```python
from build123d import *

# Parameters (mm, degrees)
BOSS_EXTRUDE1_DEPTH      = 36
BOSS_EXTRUDE1_DEPTH_BACK = 50.5
SKETCH1_R                = 12
SKETCH6_R                = 22.5
BOSS_EXTRUDE6_DEPTH      = 10.5
BOSS_EXTRUDE7_START      = 10
SKETCH7_R                = 22.5
BOSS_EXTRUDE7_DEPTH      = 10
SKETCH2_R                = 6.75
BOSS_EXTRUDE2_DEPTH      = 12
SKETCH3_R                = 107.5
BOSS_EXTRUDE3_DEPTH      = 10
SKETCH5_R                = 15
BOSS_EXTRUDE5_DEPTH      = 5
SKETCH4_R                = 6.75
BOSS_EXTRUDE4_DEPTH      = 12


with BuildPart() as part:
    # Sketch1 → Boss-Extrude1 (new, two sides: drawn at the far end of the back side and taken through both)
    with BuildSketch(Plane.XY.offset(-BOSS_EXTRUDE1_DEPTH_BACK)):
        Circle(SKETCH1_R)
    extrude(amount=BOSS_EXTRUDE1_DEPTH + BOSS_EXTRUDE1_DEPTH_BACK)

    # Sketch6 → Boss-Extrude6 (add)
    with BuildSketch(Plane(origin=(0, 0, -50.5), x_dir=(-1, 0, 0), z_dir=(0, 0, -1))):
        with Locations(Location((0, 0, 0), (0, 0, 180))):
            Circle(SKETCH6_R)
    extrude(amount=BOSS_EXTRUDE6_DEPTH)

    # Sketch7 → Boss-Extrude7 (add)
    with BuildSketch(Plane.XY.offset(36).offset(BOSS_EXTRUDE7_START)):
        Circle(SKETCH7_R)
    extrude(amount=-BOSS_EXTRUDE7_DEPTH)

    # Sketch2 → Boss-Extrude2 (add)
    with BuildSketch(Plane(origin=(0, 0, -61), x_dir=(-1, 0, 0), z_dir=(0, 0, -1))):
        with BuildLine():
            Line((-7.5, -190), (7.5, -190))
            ThreePointArc((7.5, -190), (14.571067812, -187.071067812), (17.5, -180))
            Line((17.5, -180), (17.5, 20))
            ThreePointArc((17.5, 20), (14.571067812, 27.071067812), (7.5, 30))
            Line((7.5, 30), (-7.5, 30))
            ThreePointArc((-7.5, 30), (-14.571067812, 27.071067812), (-17.5, 20))
            Line((-17.5, 20), (-17.5, -180))
            ThreePointArc((-17.5, -180), (-14.571067812, -187.071067812), (-7.5, -190))
        make_face()
        with Locations((0, -170)):
            Circle(SKETCH2_R, mode=Mode.SUBTRACT)
    extrude(amount=BOSS_EXTRUDE2_DEPTH)

    # Sketch3 → Boss-Extrude3 (add)
    with BuildSketch(Plane.XY.offset(46)):
        Circle(SKETCH3_R)
        with BuildLine():
            Line((0, 30), (0, 90))
            ThreePointArc((0, 90), (45, 77.942286341), (77.942286341, 45))
            Line((77.942286341, 45), (25.980762114, 15))
            ThreePointArc((25.980762114, 15), (15, 25.980762114), (0, 30))
        make_face(mode=Mode.SUBTRACT)
        with BuildLine():
            Line((28.531695489, 9.270509831), (85.595086467, 27.811529494))
            ThreePointArc((85.595086467, 27.811529494), (88.033284066, -18.712052174), (66.883034293, -60.221754572))
            Line((66.883034293, -60.221754572), (22.294344764, -20.073918191))
            ThreePointArc((22.294344764, -20.073918191), (29.344428022, -6.237350725), (28.531695489, 9.270509831))
        make_face(mode=Mode.SUBTRACT)
        with BuildLine():
            Line((17.633557569, -24.270509831), (52.900672706, -72.811529494))
            ThreePointArc((52.900672706, -72.811529494), (9.407561694, -89.506970583), (-36.606297877, -82.219091188))
            Line((-36.606297877, -82.219091188), (-12.202099292, -27.406363729))
            ThreePointArc((-12.202099292, -27.406363729), (3.135853898, -29.835656861), (17.633557569, -24.270509831))
        make_face(mode=Mode.SUBTRACT)
        with BuildLine():
            Line((-17.633557569, -24.270509831), (-52.900672706, -72.811529494))
            ThreePointArc((-52.900672706, -72.811529494), (-82.219091188, -36.606297877), (-89.506970583, 9.407561694))
            Line((-89.506970583, 9.407561694), (-29.835656861, 3.135853898))
            ThreePointArc((-29.835656861, 3.135853898), (-27.406363729, -12.202099292), (-17.633557569, -24.270509831))
        make_face(mode=Mode.SUBTRACT)
        with BuildLine():
            Line((-28.531695489, 9.270509831), (-85.595086467, 27.811529494))
            ThreePointArc((-85.595086467, 27.811529494), (-60.221754572, 66.883034293), (-18.712052174, 88.033284066))
            Line((-18.712052174, 88.033284066), (-6.237350725, 29.344428022))
            ThreePointArc((-6.237350725, 29.344428022), (-20.073918191, 22.294344764), (-28.531695489, 9.270509831))
        make_face(mode=Mode.SUBTRACT)
    extrude(amount=BOSS_EXTRUDE3_DEPTH)

    # Sketch5 → Boss-Extrude5 (add)
    with BuildSketch(Plane.XY.offset(56)):
        Circle(SKETCH5_R)
    extrude(amount=BOSS_EXTRUDE5_DEPTH)

    # Sketch4 → Boss-Extrude4 (add)
    with BuildSketch(Plane.XY.offset(61)):
        with BuildLine():
            Line((-7.5, -30), (7.5, -30))
            ThreePointArc((7.5, -30), (14.571067812, -27.071067812), (17.5, -20))
            Line((17.5, -20), (17.5, 180))
            ThreePointArc((17.5, 180), (14.571067812, 187.071067812), (7.5, 190))
            Line((7.5, 190), (-7.5, 190))
            ThreePointArc((-7.5, 190), (-14.571067812, 187.071067812), (-17.5, 180))
            Line((-17.5, 180), (-17.5, -20))
            ThreePointArc((-17.5, -20), (-14.571067812, -27.071067812), (-7.5, -30))
        make_face()
        with Locations((0, 170)):
            Circle(SKETCH4_R, mode=Mode.SUBTRACT)
    extrude(amount=BOSS_EXTRUDE4_DEPTH)


solid = part.part
```
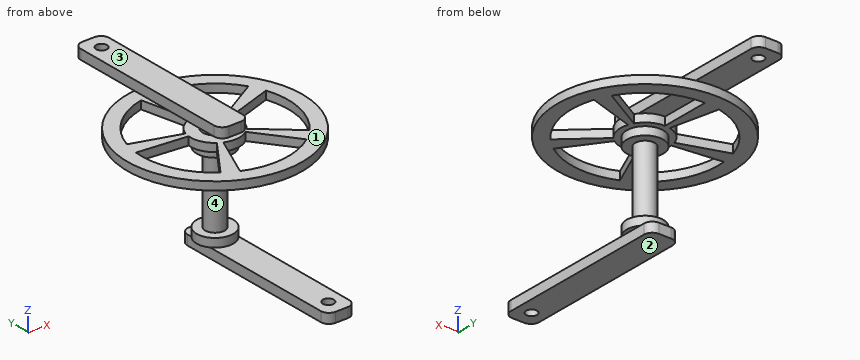
Geometry: final body of the model. Coordinates: model frame, mm. Face numbers are marked on the shaded views. Coordinates: 2 decimals unless noted, no trailing zeros. Order: outer loops, then holes, each group sorted by start corner. A loop starts at its lowest first (then second) coordinate and runs counter-clockwise, first axis right, second up. Notation, with made-up numbers: (68.25, 55) -> (127.25, 55) arc R22 cw to (127.25, 65) -> close; hole circle Ø3 at (-25.75, 2.25). An arc over 180 degrees is marked (long way). Write item = value, one per line.
(1) Cut plane B-B on y = -170. Return loops of the section in (x, z).
Solved:
outline = (-17.5, -73) -> (-6.75, -73) -> (-6.75, -61) -> (-17.5, -61) -> close; (6.75, -73) -> (17.5, -73) -> (17.5, -61) -> (6.75, -61) -> close
(2) Cut plane D-D on z = 12. Return loops of the section in (x, y), plus the area to 3 significant figures.
Solved:
outline = circle Ø24 at (0, 0)
area = 452 mm²
(3) Line query: line 1 (Z direction, x = 11.5, y = -22.5); line 2 (Y direction, x = 0, z = -67); line 3 (Z direction, x = 1, y = 130). Output: solid intervals per line, ascending.
Solved:
line_1 = -73 to -61, 46 to 56, 61 to 73
line_2 = -190 to -176.75, -163.25 to 30
line_3 = 61 to 73
(4) Cut plane A-A on x = -59. Return loops of the section in (y, z).
Solved:
outline = (-89.86, 46) -> (-67.96, 46) -> (-67.96, 56) -> (-89.86, 56) -> close; (6.2, 46) -> (19.17, 46) -> (19.17, 56) -> (6.2, 56) -> close; (67.96, 46) -> (89.86, 46) -> (89.86, 56) -> (67.96, 56) -> close
(5) Pull-direction query (Z, two-part tool) for the marked faces 1, 2, 3 and 4; classes: pulls with the +Z half, pulls with the -Z half, needs draft (parallel to the pull), parting line crosses it, or undercut.
Solved:
face_1 = undercut
face_2 = pulls with the -Z half
face_3 = pulls with the +Z half
face_4 = undercut
(6) Pin query (flat end, axial travel): pin 1 Ø12 at (x, y) = (-57, 94) entering from +Z; pin 2 Ø17.5 at (x, y) = (5, -81) entering from +Z; pin 3 Ø2.5 at (x, y) = (-20, -5) entering from -Z; pin 4 Ø10 at (x, y) = (-47.5, -104.5) entering from +Z. Return the tip coordinate at first contact, or that it passes through.
Solved:
pin_1 = 56
pin_2 = -61
pin_3 = -61
pin_4 = through
(7) Cut plane C-C on y = 63. Return loops of the section in (x, z), plus the area to 3 significant figures.
Solved:
outline = (-87.1, 46) -> (-64.27, 46) -> (-64.27, 56) -> (-87.1, 56) -> close; (-17.5, 61) -> (17.5, 61) -> (17.5, 73) -> (-17.5, 73) -> close; (-13.39, 46) -> (0, 46) -> (0, 56) -> (-13.39, 56) -> close; (64.27, 46) -> (87.1, 46) -> (87.1, 56) -> (64.27, 56) -> close
area = 1,010 mm²
